Here's the drawing with two shaded views (mm, measured from the low corner). I have some questions. Give positions to 0.01 mm unless a question says otherwise; leave off trailing zeros. Write each loop counter-clockwise with the first axis right and the second up, starting at its lowest first coordinate (ties: lowest second). Pieces come first, ordered by that corner, then holes. Notation, with made-up numbers: (15, 26.25) - (39, 26.25) arc R23 cw to (39, 52.25) - close; hole circle Ø3 at (-8.75, -32). An arc over 180 degrees is marked (long way). Answer as a JSON object with one key per item and string values. Group by question number.
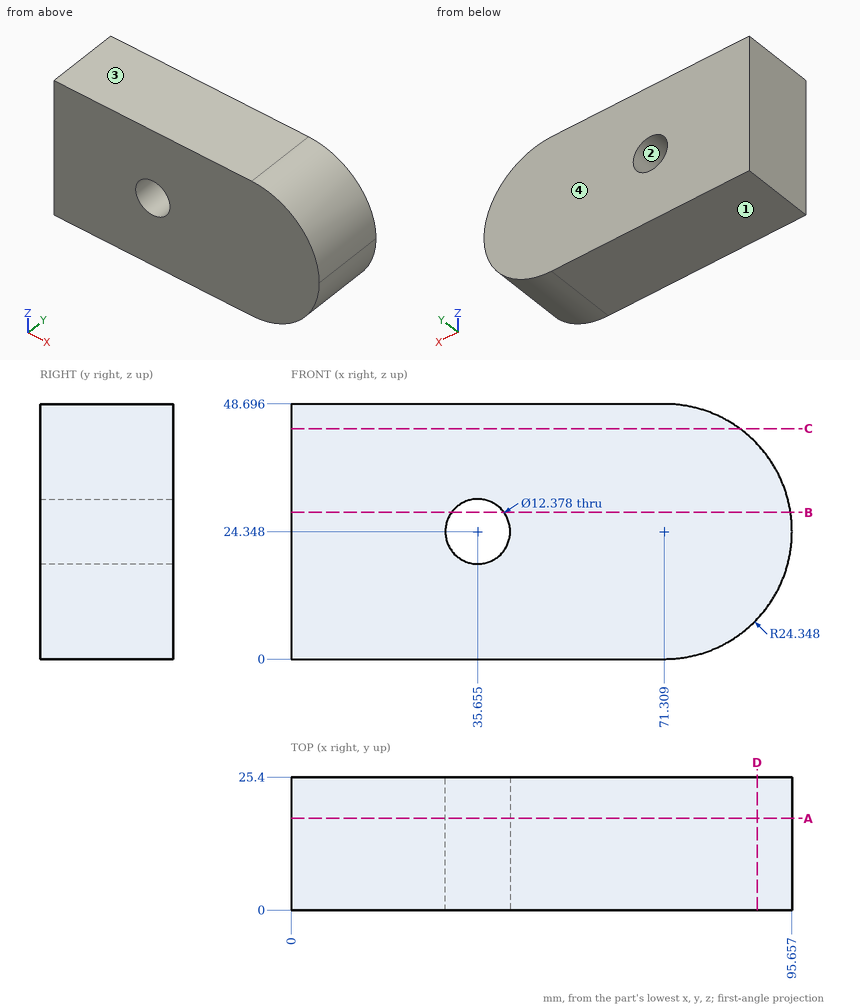
(1) If we mould it in two halves opening along Z, with no side actions, what happens to the marked faces 1, 2, 3 and 4? For each: +Z half, -Z half, draft (parallel to the pull), parting line (faces both ways), or undercut.
(2) I want a section at D-D, the plane x = 89. Please give me the cut outline in (y, z), and give its area (3 significant figures).
(3) I want a section at A-A, the plane y = 17.5. Please give me the cut outline in (x, z) (1 decimal).
(4) I need wall thicknesses on L1, parallel to X at y = 7.5, z = 29 (1 decimal); L2, parallel to X at y = 7, z = 25; L3, parallel to Z at x = 30, y = 1.75 (1 decimal). Which ranges of each line are inside material? Lowest first, please.
(5) I want a section at B-B, the plane z = 28. Please give me the cut outline in (x, y).
(6) Will these pins go through, and if not, where does the flat tip stop? P1, Ø5, axis at y = 19, z = 32, coming from the +X side; P2, Ø1.5, axis at y = 21.5, z = 32.5, coming from the +X side (1 decimal).
(7) I want a section at C-C, the plane z = 44. Please give me the cut outline in (x, y).
Entries:
{
 "1": {"face 1": "-Z half", "face 2": "undercut", "face 3": "+Z half", "face 4": "draft"},
 "2": {"outline": "(0, 7.62) - (25.4, 7.62) - (25.4, 41.08) - (0, 41.08) - close", "area": "850 mm^2"},
 "3": {"outline": "(0, 0) - (71.3, 0) arc R24.3 ccw to (95.7, 24.3) arc R24.3 ccw to (71.3, 48.7) - (0, 48.7) - close; hole circle Ø12.4 at (35.7, 24.3)"},
 "4": {"L1": "0 to 31.6, 39.7 to 95.2", "L2": "0 to 29.5, 41.81 to 95.65", "L3": "0 to 21.8, 26.9 to 48.7"},
 "5": {"outline": "(0, 0) - (30.66, 0) - (30.66, 25.4) - (0, 25.4) - close; (40.65, 0) - (95.38, 0) - (95.38, 25.4) - (40.65, 25.4) - close"},
 "6": {"P1": "x = 95.11", "P2": "x = 94.5"},
 "7": {"outline": "(0, 0) - (85.68, 0) - (85.68, 25.4) - (0, 25.4) - close"}
}
